For this review, take the finished solid that the model builds, in its own axes (mm). A direction names the side the tool comes from. Round coordinates to 2 decimals unless told otherwise and drop trailing zeros. Loops run counter-clockwise (first coordinate to the right, second up) from the corner with the lowest first, then second, coordinate; pieces in that order, holes last.
1) Mouldability with a two-part tool opening along X and no side actions: class faces 3 (the cylindrical face through (-134.91, 103.44, 28.24)), 4 (the cylindrical face through (108.456, 100.291, 18.252)), 5 (the flat face through (-39, -125, 47)) as pulls with the +X half, pulls with the -X half, needs draft (parallel to the pull), parting line crosses it, or undercut.
2) Take a section at B-B (y = 61). State the section outline as (x, z) points.
3) Take a section at C-C (z = 42.5). Give the number of separate pieces and of enclosed holes in the cut face, then the cut area to 3 significant figures.
4) Tool access review of faces 1 (the flat face through (4, 155, 36)), 2 (the cylindrical face through (144.455, -2.884, 18.252)): name each direction out of +Z, -Z, +X, -X, +Y, -Y from which nothing blocks a thin tool from reaching the whole face with its end or side.
5) Wall thickness on L1, parallel to Y at x = 0, z = 23; L2, parallel to Y at x = 0, z = 43.5; L3, parallel to X at y = 108, z = 31.5: over which ranges is each line inside the solid? List them lowest first.
6) Take a section at A-A (x = 0). State the section outline as (y, z) points, then the cut area to 3 significant figures.
7) Insertion check: pin 1 (10 mm diameter, centred on x = 107, y = 103.5, fed in from +Z); pin 2 (4 mm diameter, centred on x = -44.5, z = 14, fed in from +Y); pin 3 (10 mm diameter, centred on x = -125.5, z = 37, fed in from -Y). Each pin has a flat end and moves straight along its axis. Give the tip position at first contact, or say it passes through.
8) Take a section at D-D (x = 72). State the section outline as (y, z) points.
Autodesk Inventor part; units mm, degrees
ref_plane "YZ Plane" through (0, 0, 0) normal (1, 0, 0) x (0, 1, 0)
ref_plane "XZ Plane" through (0, 0, 0) normal (0, 1, 0) x (-1, 0, 0)
ref_plane "XY Plane" through (0, 0, 0) normal (0, 0, 1) x (1, 0, 0)
sketch "Sketch1" plane through (0, 0, 0) normal (0, 0, 1) x (1, 0, 0)
  circle A0 centre (0, 0) radius 130
  circle A1 centre (0, 0) radius 170
  dimension "d0" = 40
  dimension "d1" = 260
extrude "Extrusion1" add sketch "Sketch1" along normal blind 47
sketch "Sketch2" plane through (0, 0, 47) normal (0, 0, 1) x (1, 0, 0)
  circle A0 centre (0, 0) radius 170 construction
  circle A1 centre (0, 0) radius 130 construction
  line L0 (0, 170) -> (0, 130) construction
  circle A2 centre (0, 150) radius 6.25
  dimension "d4" = 12.5
extrude "Extrusion2" cut sketch "Sketch2" against normal through all
sketch "Sketch3" plane through (0, 0, 47) normal (0, 0, 1) x (1, 0, 0)
  circle A0 centre (0, 150) radius 6.25
  circle A1 centre (0, 150) radius 10
  point P0 (0, 0)
  dimension "d10" = 20
extrude "Extrusion3" cut sketch "Sketch3" against normal blind 11
pattern_circular "Circular Pattern1" count 8 over 360 about axis through (0, 0, 0) along (0, 0, 1) of "Extrusion2", "Extrusion3"
sketch "Sketch4" plane through (0, 0, 0) normal (0, 0, -1) x (-1, 0, 0)
  circle A0 centre (0, 0) radius 170
  circle A1 centre (0, 0) radius 175
  dimension "d13" = 5
extrude "Extrusion4" add sketch "Sketch4" against normal blind 10
equation "\"d1\" = Вал_ось_диаметр_НОС"
equation "\"d2\" = Барабан_толщина_посад_кольца"
properties part number "ДМС 102 Опорное кольцо вала перед ПВГ"
Response:
1. face 3: parting line crosses it
1. face 4: undercut
1. face 5: needs draft
2. outline: (-164.02, 0) - (-114.8, 0) - (-114.8, 47) - (-158.68, 47) - (-158.68, 10) - (-164.02, 10) - close; (114.8, 0) - (164.02, 0) - (164.02, 10) - (158.68, 10) - (158.68, 47) - (114.8, 47) - close
3. separate pieces: 1
3. enclosed holes: 9
3. area: 35,200 mm2
4. face 1: +Z
4. face 2: +Z, -Z
5. L1: y = -170 to -156.25, -143.75 to -130, 130 to 143.75, 156.25 to 170
5. L2: y = -170 to -160, -140 to -130, 130 to 140, 160 to 170
5. L3: x = -131.29 to -112.01, -100.12 to -72.36, 72.36 to 100.12, 112.01 to 131.29
6. outline: (-175, 0) - (-156.25, 0) - (-156.25, 36) - (-160, 36) - (-160, 47) - (-170, 47) - (-170, 10) - (-175, 10) - close; (-143.75, 0) - (-130, 0) - (-130, 47) - (-140, 47) - (-140, 36) - (-143.75, 36) - close; (130, 0) - (143.75, 0) - (143.75, 36) - (140, 36) - (140, 47) - (130, 47) - close; (156.25, 0) - (175, 0) - (175, 10) - (170, 10) - (170, 47) - (160, 47) - (160, 36) - (156.25, 36) - close
6. area: 2,520 mm2
7. pin 1: stops at z = 36
7. pin 2: stops at y = 164.6
7. pin 3: stops at y = -119.92
8. outline: (-159.5, 0) - (-108.24, 0) - (-108.24, 47) - (-154, 47) - (-154, 10) - (-159.5, 10) - close; (108.24, 0) - (159.5, 0) - (159.5, 10) - (154, 10) - (154, 47) - (108.24, 47) - close
